The figure shows three views and two pictorial views of one solid part (mm, origin at its lowest corner). Answer the questions. Coordinates: 2 decimals unless noted, no trailing zeros. Write each loop counter-clockwise with the first axis right and the second up, starting at its lowest first coordinate (ties: lowest second). Pieces come first, ordered by that corner, then holes.
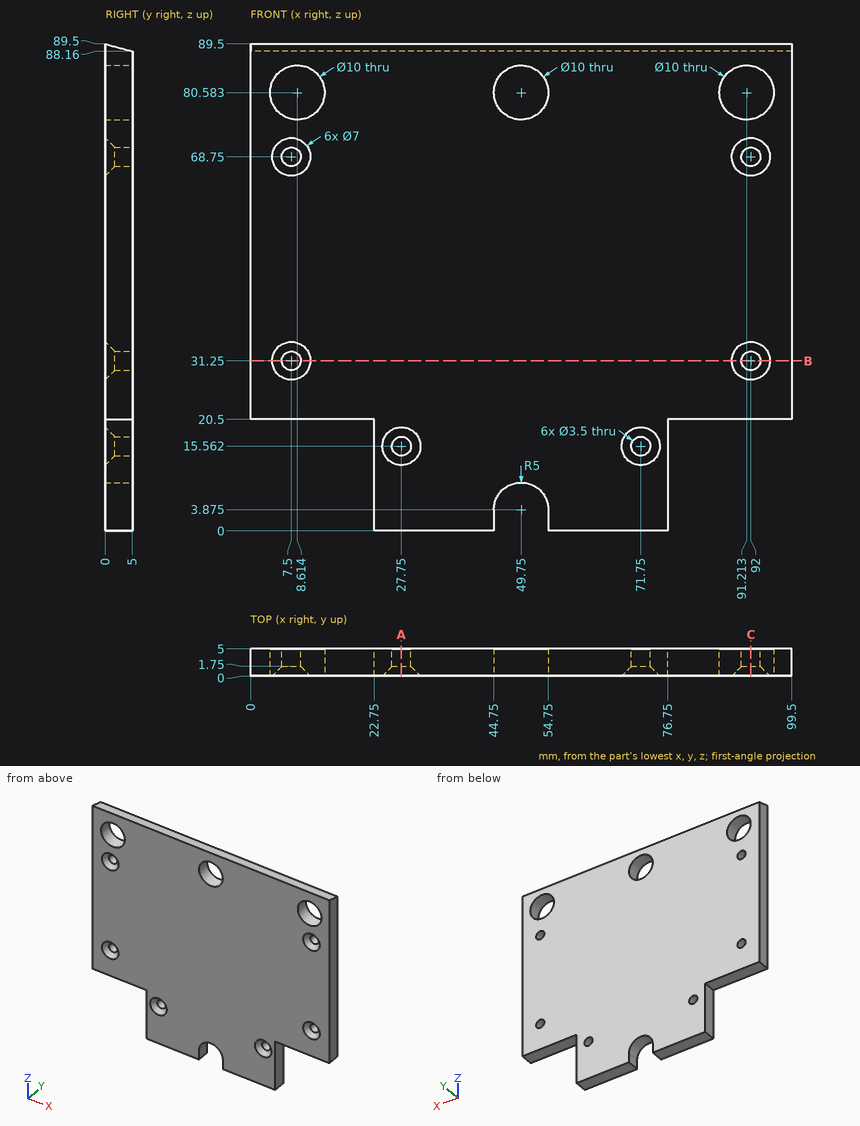
Q1. The part is cut by section A-A, the plane x = 27.75. Write down the section's boundary in (y, z).
Answers below:
outline: (0, 0) - (5, 0) - (5, 13.81) - (1.75, 13.81) - (0, 12.06) - close; (0, 19.06) - (1.75, 17.31) - (5, 17.31) - (5, 88.16) - (0, 89.5) - close
Q2. Given pin 1 (4.5 mm diameter, centred on x = 27.75, z = 15.56, fed in from -Y); pin 2 (2 mm diameter, centred on x = 71.75, z = 15.56, fed in from -Y); pin 3 (3 mm diameter, centred on y = 1.5, z = 1.5, fed in from -X); pin 4 (3 mm diameter, centred on y = 3.5, z = 1, fed in from +X), each flat-ended and moving along its own axis, determine where each tip first touches the part or whether it passes through.
Answers below:
pin 1: stops at y = 1.25
pin 2: passes through
pin 3: stops at x = 22.75
pin 4: stops at x = 76.75
Q3. The part is cut by section C-C, the plane x = 92. State how many separate pieces and enclosed holes the cut face has, then the cut area to 3 significant figures.
Answers below:
separate pieces: 4
enclosed holes: 0
area: 251 mm2
Q4. Find the intervals of material crossed by probe 1 along X at (y, z) = (2.65, 31.25); probe 2 along Z at (x, y) = (7.5, 3.5); probe 3 along Z at (x, y) = (7.5, 2.85) (1 decimal), in increasing order.
Answers below:
probe 1: x = 0 to 5.75, 9.25 to 90.25, 93.75 to 99.5
probe 2: z = 20.5 to 29.5, 33 to 67, 70.5 to 75.71, 85.46 to 88.56
probe 3: z = 20.5 to 29.5, 33 to 67, 70.5 to 75.7, 85.5 to 88.7
Q5. The part is cut by section B-B, the plane z = 31.25. Write down the section's boundary in (x, y).
Answers below:
outline: (0, 0) - (4, 0) - (5.75, 1.75) - (5.75, 5) - (0, 5) - close; (9.25, 1.75) - (11, 0) - (88.5, 0) - (90.25, 1.75) - (90.25, 5) - (9.25, 5) - close; (93.75, 1.75) - (95.5, 0) - (99.5, 0) - (99.5, 5) - (93.75, 5) - close
